```python
from build123d import *

# Parameters (mm, degrees)
BOSS_EXTRUDE4_DEPTH = 19.05
CUT_EXTRUDE5_DEPTH  = 9.525
CUT_EXTRUDE6_DEPTH  = 9.525
SKETCH10_R          = 3.175
CUT_EXTRUDE7_DEPTH  = 19.05


with BuildPart() as part:
    # Sketch2 → Boss-Extrude4 (new body)
    with BuildSketch(Plane(origin=(0, 0, 0), x_dir=(1, 0, 0), z_dir=(0, 1, 0))):
        Polygon((-183.626593256, 296.748681841), (-193.321682542, 313.147088585), (-226.11849603, 293.756910013), (-52.443119188, 0), (-29.917583168, -38.1), (394.367218256, -755.741121604), (427.164031744, -736.350943032), (0, -13.839851848), (-8.182416832, 0), align=None)
    extrude(amount=BOSS_EXTRUDE4_DEPTH)

    # Sketch8 → Cut-Extrude5 (cut)
    with BuildSketch(Plane(origin=(0, 19.05, 0), x_dir=(1, 0, 0), z_dir=(0, 1, 0))):
        Polygon((-193.321682542, 313.147088585), (-215.267964049, 300.171976915), (-221.216787177, 285.466092555), (-196.814123155, 244.191092555), (-178.833212823, 288.641092555), align=None)
    extrude(amount=-CUT_EXTRUDE5_DEPTH, mode=Mode.SUBTRACT)

    # Sketch9 → Cut-Extrude6 (cut)
    with BuildSketch(Plane.XZ):
        Polygon((-52.443119188, 0), (-29.917583168, 38.1), (0, 38.1), (0, 13.839851848), (-8.182416832, 0), align=None)
    extrude(amount=-CUT_EXTRUDE6_DEPTH, mode=Mode.SUBTRACT)

    # Sketch10 → Cut-Extrude7 (cut)
    with BuildSketch(Plane.XZ):
        with Locations(Location((-200.025, -287.053592555, 0), (0, 0, 270))):
            Circle(SKETCH10_R)
        with Locations(Location((-19.05, 19.05, 0), (0, 0, 270))):
            Circle(SKETCH10_R)
    extrude(amount=-CUT_EXTRUDE7_DEPTH, mode=Mode.SUBTRACT)


solid = part.part
```
The listing builds one solid part. Answer for the finished solid, in the listing's coordinates (mm). Give positions to 0.01 mm unless a question says otherwise; leave off trailing zeros. Write each loop counter-clockwise with the first axis right and the second up, starting at its lowest first coordinate (ties: lowest second). Pieces come first, ordered by that corner, then holes. Notation, with made-up numbers: (51, -35) - (57, -35) arc R29 ccw to (57, 2) - close; hole circle Ø11 at (17, 69.5). An arc over 180 degrees is marked (long way). Use one line per item in the form item = value. Start each with the question number.
1) Find section B-B on z = 573.5. Determine the outline of the cut face in (x, y), plus the area to 3 significant figures.
2) Flat-ended cylindrical pins translate along their axes: pin 1 Ø6 at (x, y) = (158, 5) entering from -Z; pin 2 Ø8 at (y, z) = (14.5, 483.5) entering from -X; pin 3 Ø1.5 at (x, y) = (255, 2) entering from -Z; pin 4 Ø8.5 at (x, z) = (-19.05, 19.05) entering from +Y. Find the tip coordinate at first contact, or state that the pin passes through.
3) Find section A-A on x = 215. Determine the outline of the cut face in (y, z), plus the area to 3 significant figures.
4) Consider line 1 along X through (y, z) = (13.5, 19.05) (3 decimals); line 2 along Z through (x, y) = (77, 3.25); line 3 along Z through (x, y) = (-36.5, 3.25). Determine where each line is inside the solid, lowest interval first. Write a range as from..to.
5) The mould has two halves that part along Z. Classify faces 1 (the face through (-200, 9.525, -279)), 2 (the face through (-213.135, 7.275, -301.433)), 3 (the face through (410.54, 9.39, 746.18)), 4 (the face through (-20, 9.525, 15)): pulls with the +Z half, pulls with the -Z half, needs draft (parallel to the pull), parting line crosses it, or undercut.
Geometry results:
q1.outline = (286.62, 0) - (330.88, 0) - (330.88, 19.05) - (286.62, 19.05) - close
q1.area = 843 mm2
q2.pin_1 = 276.01
q2.pin_2 = 231.05
q2.pin_3 = 443.88
q2.pin_4 = 19.05
q3.outline = (0, 377.49) - (19.05, 377.49) - (19.05, 452.36) - (0, 452.36) - close
q3.area = 1,430 mm2
q4.line_1 = -41.18..-22.225, -15.875..3.08
q4.line_2 = 144.08..218.94
q4.line_3 = -47.9..0
q5.face_1 = needs draft
q5.face_2 = pulls with the -Z half
q5.face_3 = pulls with the +Z half
q5.face_4 = undercut
